Part model, mm, in its own coordinate system. Face numbers are marked on the shaded views. A direction names the side the tool comes from. Give positions to 0.01 mm unless a question says otherwise; leave off trailing zeros. Write each loop counter-clockwise with the first axis right and the second up, starting at its lowest first coordinate (ties: lowest second). Pieces come first, ordered by that corner, then holes. Notation, with made-up numbers: M 5,-32.5 L 53,-32.5 A8 cw 53,-24.5 Z; hole C 15.5,-26.75 d1. An arc over 180 degrees is marked long. Use a Markdown table: item, result.
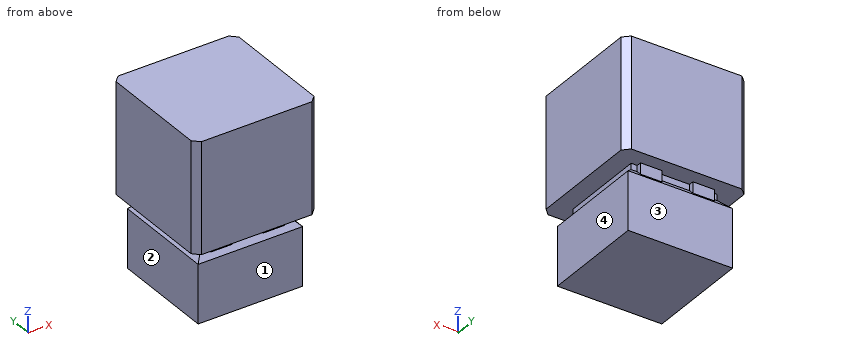
```python
from build123d import *

# Parameters (mm, degrees)
BOX005_W        = 20
BOX005_H        = 20
BOX005_DEPTH    = 18
CHAMFER003_SIZE = 1
BOX004_W        = 17
BOX004_H        = 17
BOX004_DEPTH    = 11
CHAMFER002_SIZE = 1.5
BOX003_W        = 14
BOX003_H        = 14
BOX003_DEPTH    = 1
BOX008_W        = 3.5
BOX008_H        = 1
BOX008_DEPTH    = 2
BOX007_W        = 3.5
BOX007_H        = 1
BOX007_DEPTH    = 2
BOX006_W        = 3.5
BOX006_H        = 1
BOX006_DEPTH    = 2
BOX009_W        = 3.5
BOX009_H        = 1
BOX009_DEPTH    = 2


with BuildPart() as chamfer003:
    # Box005 → Box005 (new body)
    with BuildSketch(Plane(origin=(-10, -10, 12), x_dir=(1, 0, 0), z_dir=(0, 0, 1))):
        with Locations((10, 10)):
            Rectangle(BOX005_W, BOX005_H)
    extrude(amount=BOX005_DEPTH)

    # Chamfer003
    chamfer003_edges = [chamfer003.edges().sort_by_distance(p)[0] for p in [
        (-10, -10, 21),
        (-10, 10, 21),
        (10, -10, 21),
        (10, 10, 21),
    ]]
    chamfer(chamfer003_edges, length=CHAMFER003_SIZE)


with BuildPart() as chamfer002:
    # Box004 → Box004 (new body)
    with BuildSketch(Plane(origin=(-8.5, -8.5, 0), x_dir=(1, 0, 0), z_dir=(0, 0, 1))):
        with Locations((8.5, 8.5)):
            Rectangle(BOX004_W, BOX004_H)
    extrude(amount=BOX004_DEPTH)

    # Chamfer002
    chamfer002_edges = [chamfer002.edges().sort_by_distance(p)[0] for p in [
        (-8.5, 0, 11),
        (8.5, 0, 11),
        (0, -8.5, 11),
        (0, 8.5, 11),
    ]]
    chamfer(chamfer002_edges, length=CHAMFER002_SIZE)


with BuildPart() as cube003:
    # Box003 → Box003 (new body)
    with BuildSketch(Plane(origin=(-7, -7, 11), x_dir=(1, 0, 0), z_dir=(0, 0, 1))):
        with Locations((7, 7)):
            Rectangle(BOX003_W, BOX003_H)
    extrude(amount=BOX003_DEPTH)


with BuildPart() as cube008:
    # Box008 → Box008 (new body)
    with BuildSketch(Plane(origin=(2.5, 6.8, 10), x_dir=(1, 0, 0), z_dir=(0, 0, 1))):
        with Locations((1.75, 0.5)):
            Rectangle(BOX008_W, BOX008_H)
    extrude(amount=BOX008_DEPTH)


with BuildPart() as cube007:
    # Box007 → Box007 (new body)
    with BuildSketch(Plane(origin=(2.5, -7.8, 10), x_dir=(1, 0, 0), z_dir=(0, 0, 1))):
        with Locations((1.75, 0.5)):
            Rectangle(BOX007_W, BOX007_H)
    extrude(amount=BOX007_DEPTH)


with BuildPart() as cube006:
    # Box006 → Box006 (new body)
    with BuildSketch(Plane(origin=(-6, -7.8, 10), x_dir=(1, 0, 0), z_dir=(0, 0, 1))):
        with Locations((1.75, 0.5)):
            Rectangle(BOX006_W, BOX006_H)
    extrude(amount=BOX006_DEPTH)


with BuildPart() as button_slot:
    # Box009 → Box009 (new body)
    with BuildSketch(Plane(origin=(-6, 6.8, 10), x_dir=(1, 0, 0), z_dir=(0, 0, 1))):
        with Locations((1.75, 0.5)):
            Rectangle(BOX009_W, BOX009_H)
    extrude(amount=BOX009_DEPTH)

    # Fusion: union Cube008, Cube007, Cube006
    add(cube008.part)
    add(cube007.part)
    add(cube006.part)

    # Fusion001: union Chamfer003, Chamfer002, Cube003
    add(chamfer003.part)
    add(chamfer002.part)
    add(cube003.part)


solid = button_slot.part
```
1. Drop flat-ended pins along their axis: P1, Ø0.9, axis at y = -7.5, z = 11.5, coming from the -X side; P2, Ø3, axis at x = 0, z = 2.5, coming from the +Y side; P3, Ø0.9, axis at y = 7.5, z = 11, coming from the +X side. Give the stop position or say it passes through.
Findings below:
| item | result |
|---|---|
| P1 | x = -6 |
| P2 | y = 8.5 |
| P3 | x = 7.45 |
2. Tool access for the marked faces 1, 2, 3 and 4: list every direction of +Z, -Z, +X, -X, +Y, -Y with a clear straight run to the whole face (end or side of a thin tool).
Findings below:
| item | result |
|---|---|
| face 1 | -Z, +X, -X, -Y |
| face 2 | -Z, -X, +Y, -Y |
| face 3 | -Z, +X, -X, +Y |
| face 4 | -Z, +X, +Y, -Y |
3. Cut at D-D, the plane z = 8.25. Give the cut face in (x, y), then the cut area to 3 significant figures.
Findings below:
| item | result |
|---|---|
| outline | M -8.5,-8.5 L 8.5,-8.5 L 8.5,8.5 L -8.5,8.5 Z |
| area | 289 mm2 |
4. Drill centre lines: L1, parallel to Z at x = -8, y = 0.25; L2, parallel to Y at x = -5.5, z = 4.5. Where is each one in solid material? Low to high.
Findings below:
| item | result |
|---|---|
| L1 | 0 to 10, 12 to 30 |
| L2 | -8.5 to 8.5 |
5. Cut at A-A, the plane x = 7.5. Give the cut face in (y, z).
Findings below:
| item | result |
|---|---|
| outline | M -10,12 L 10,12 L 10,30 L -10,30 Z; M -8.5,0 L 8.5,0 L 8.5,9.5 L 7.5,10.5 L -7.5,10.5 L -8.5,9.5 Z |
6. Cut at B-B, the plane y = -5.5. Give the cut face in (x, z), then the cut area to 3 significant figures.
Findings below:
| item | result |
|---|---|
| outline | M -10,12 L -7,12 L -7,11 L -8.5,9.5 L -8.5,0 L 8.5,0 L 8.5,9.5 L 7,11 L 7,12 L 10,12 L 10,30 L -10,30 Z |
| area | 559 mm2 |
